Geometry: final body of the model. Coordinates: model frame, mm. Face numbers are marked on the shaded views. A direction names the side the tool comes from. Give positions to 0.01 mm unless a question says otherwise; leave off trailing zeros. Write each loop counter-clockwise with the first axis right and the second up, starting at its lowest first coordinate (ties: lowest second). Pieces come first, ordered by that corner, then holes. Notation, with made-up numbers: M 29,3.5 L 47,3.5 A7 ccw 47,12.5 Z; hole C 51.25,72 d8. An arc over 180 degrees is marked long. Use one line per item in the form item = value. Start each with the question number.
Item 1: Section query A-A on x = -15. Return loops of the section in (y, z).
Item 2: Material intervals for line 1 along X through (y, z) = (4, 4); line 2 along Y through (x, z) = (7, 7.5); line 3 along Y through (x, z) = (14, 7.25), sorted ascending. Write a range as from..to.
Item 3: Section query C-C on y = -19. Return loops of the section in (x, z).
Item 4: Access query for the marked faces 5, 6, 7, 8 and 9. Directions: +Z, -Z, +X, -X, +Y, -Y. A direction counts if a zero-diameter tool reaches every point of the face in a straight line with its end or side. Return the directions, or none.
Item 5: Pull-direction query (Y, two-part tool) for the marked faces 1, 2, 3 and 4; classes: released by +Y, released by -Y, zero draft, split by the parting line, or undercut.
Item 6: Contact query for flat-ended pins moving along their axis: P1, Ø1.8, axis at y = -19.5, z = 4, coming from the +X side; P2, Ø1, axis at y = -14.5, z = 1.5, coming from the +X side; P3, Ø1.2, axis at x = 13.5, z = 2, coming from the +Y side; P4, Ø4, axis at y = 8, z = 6, coming from the +X side. Output: stop coordinate, or through.
Item 7: Section query B-B on z = 3. Return loops of the section in (x, y), then the cut area to 3 significant figures.
from build123d import *

# Parameters (mm, degrees)
F1_DEPTH = 2
F3_DEPTH = 6
F4_W     = 24
F4_H     = 6
F5_DEPTH = 1
F6_R     = 1
F8_DEPTH = 10


with BuildPart() as f1:
    # F0 (on Top) → F1 (new body)
    with BuildSketch(Plane.XY):
        Polygon((-24, 0), (-24, -28), (17, -28), (17, 0), (12, 0), (12, 21), (-12, 21), (-12, 0), align=None)
    extrude(amount=F1_DEPTH)

    # F2 (on face) → F3 (join)
    with BuildSketch(Plane.XY.offset(2)):
        Polygon((-24, 0), (-24, -28), (17, -28), (17, 0), (12, 0), (12, 21), (-12, 21), (-12, 0), align=None)
        Polygon((-23, -1), (-11, -1), (-11, 20), (11, 20), (11, -1), (16, -1), (16, -27), (-23, -27), align=None, mode=Mode.SUBTRACT)
    extrude(amount=F3_DEPTH)

    # F4 (on face) → F5 (cut, through all)
    with BuildSketch(Plane.YZ.offset(17)):
        with Locations((-14, 5)):
            Rectangle(F4_W, F4_H)
    extrude(amount=-F5_DEPTH, mode=Mode.SUBTRACT)

    # F6
    f6_edges = [f1.edges().sort_by_distance(p)[0] for p in [
        (-24, 0, 4),
        (-12, 21, 4),
        (12, 21, 4),
        (17, 0, 4),
        (17, -28, 4),
        (-24, -28, 4),
    ]]
    fillet(f6_edges, radius=F6_R)

    # F7 (on face) → F8 (join)
    with BuildSketch(Plane.YZ.offset(17)):
        Polygon((-26, 2), (-26, 8), (-27, 8), (-27, 0), (-1, 0), (-1, 8), (-2, 8), (-2, 2), (-2, 1.066827), (-26, 1.066827), align=None)
    extrude(amount=F8_DEPTH)


solid = f1.part
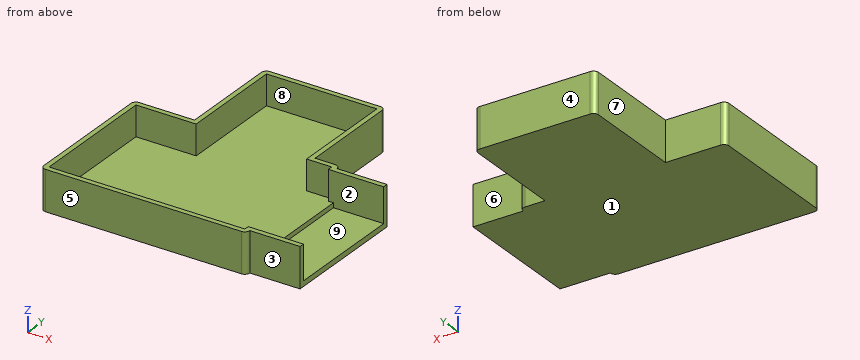
Answer sheet:
q1.outline = M -28,0 L 0,0 L 0,8 L -1,8 L -1,2 L -27,2 L -27,8 L -28,8 Z
q2.line_1 = -12..-11, 11..12
q2.line_2 = -28..-27, 20..21
q2.line_3 = -28..-27, -1..0
q3.outline = M -24,0 L 27,0 L 27,1.07 L 17,1.07 L 17,2 L -23,2 L -23,8 L -24,8 Z
q4.face_5 = +Z, -Z, +X, -X, -Y
q4.face_6 = +Z, -Z, +X, +Y
q4.face_7 = +Z, -Z, -X, +Y
q4.face_8 = +Z
q4.face_9 = +Z, +X
q5.face_1 = zero draft
q5.face_2 = undercut
q5.face_3 = released by -Y
q5.face_4 = released by +Y
q6.P1 = -23
q6.P2 = 27
q6.P3 = 0
q6.P4 = 12
q7.outline = M -24,-27 A1 ccw -23,-28 L 16,-28 A1 ccw 17,-27 L 27,-27 L 27,-26 L 16,-26 L 16,-27 L -23,-27 L -23,-1 L -11,-1 L -11,20 L 11,20 L 11,-1 L 16,-1 L 16,-2 L 27,-2 L 27,-1 L 17,-1 A1 ccw 16,0 L 12,0 L 12,20 A1 ccw 11,21 L -11,21 A1 ccw -12,20 L -12,0 L -23,0 A1 ccw -24,-1 Z
q7.area = 171 mm2
